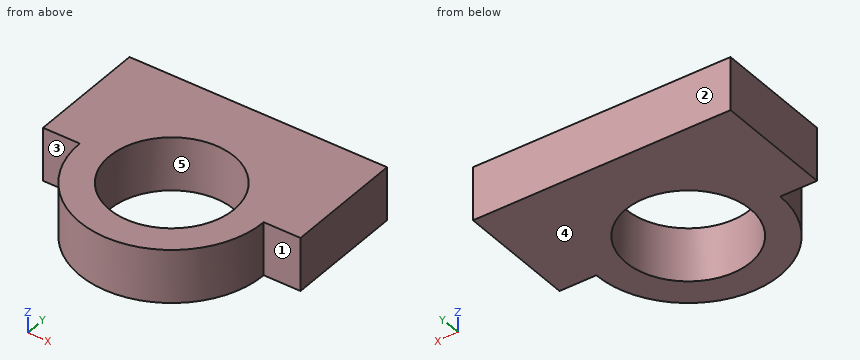
from build123d import *

# Parameters (mm, degrees)
SKETCH_1_R      = 50
SKETCH_1_R_2    = 33.9
EXTRUDE_1_DEPTH = 29


with BuildPart() as part:
    # Эскиз1 → Бобышка-Вытянуть1 (new body)
    with BuildSketch(Plane.XY):
        Circle(SKETCH_1_R)
        Circle(SKETCH_1_R_2, mode=Mode.SUBTRACT)
        with BuildLine():
            Line((70, 65), (-70, 65))
            Line((-70, 65), (-70, 0))
            Line((-70, 0), (-50, 0))
            ThreePointArc((-50, 0), (0, 50), (50, 0))
            Line((50, 0), (70, 0))
            Line((70, 0), (70, 65))
        make_face()
    extrude(amount=EXTRUDE_1_DEPTH)


solid = part.part
Build history of the part. All positions in model axes, mm. Face numbers are marked on the shaded views. A direction names the side the tool comes from. Round coordinates to 2 decimals unless told otherwise and drop trailing zeros. Write each loop counter-clockwise with the first axis right and the second up, starting at its lowest first coordinate (ties: lowest second). Pieces come first, ordered by that corner, then holes. Notation, with made-up numbers: M 60.5,-16 L 118.5,-16 A8 ccw 118.5,-2 Z; hole C 75.5,-15 d8. An arc over 180 degrees is marked long. Answer in a Markdown table with one row per item.
1. Saw through at C-C (y = 25). List the corners of the cut face in (x, z), and give its area (3 significant figures).
Geometry check:
| item | result |
|---|---|
| outline | M -70,0 L -22.9,0 L -22.9,29 L -70,29 Z; M 22.9,0 L 70,0 L 70,29 L 22.9,29 Z |
| area | 2,730 mm2 |
2. Saw through at B-B (x = 0). List the corners of the cut face in (y, z), and give its area (3 significant figures).
Geometry check:
| item | result |
|---|---|
| outline | M -50,0 L -33.9,0 L -33.9,29 L -50,29 Z; M 33.9,0 L 65,0 L 65,29 L 33.9,29 Z |
| area | 1,370 mm2 |
3. Mould opens along Y. For the marked faces 3, 4 and 5 say: +Y half, -Y half, draft (parallel to the pull), parting line (faces both ways), or undercut.
Geometry check:
| item | result |
|---|---|
| face 3 | -Y half |
| face 4 | draft |
| face 5 | undercut |
4. Which spindle directions (+Z, -Z, +X, -X, +Y, -Y) get a long thin tool onto all of the face, cutting with end or side? Do the marked faces 1 and 2. Say none if no direction does.
Geometry check:
| item | result |
|---|---|
| face 1 | +Z, -Z, +X, -Y |
| face 2 | +Z, -Z, +X, -X, +Y |
5. Probe L1, parallel to Y at x = 0, z = 13; L2, parallel to Y at x = -55, z = 4.25; L3, parallel to Y at x = 2, z = 4.5. List the from-to ranges inside material, lowest first. Write a range as [from, to].
Geometry check:
| item | result |
|---|---|
| L1 | [-50, -33.9], [33.9, 65] |
| L2 | [0, 65] |
| L3 | [-49.96, -33.84], [33.84, 65] |
6. Flat gauge pins, fed straight in: P1, Ø5, axis at y = -35.5, z = 16, coming from the +X side; P2, Ø6, axis at x = 58, z = 14, coming from the -Y side; P3, Ø1.5, axis at y = -10, z = 15, coming from the -X side. Where does each tip first touch, or does it go through?
Geometry check:
| item | result |
|---|---|
| P1 | x = 37.56 |
| P2 | y = 0 |
| P3 | x = -49.14 |
7. Saw through at D-D (x = -43.5). List the corners of the cut face in (y, z), and give its area (3 significant figures).
Geometry check:
| item | result |
|---|---|
| outline | M -24.65,0 L 65,0 L 65,29 L -24.65,29 Z |
| area | 2,600 mm2 |
8. Saw through at A-A (z = 4.25). List the corners of the cut face in (x, y).
Geometry check:
| item | result |
|---|---|
| outline | M -70,0 L -50,0 A50 ccw 50,0 L 70,0 L 70,65 L -70,65 Z; hole C 0,0 d67.8 |
